Can you work these out from the model? Positions are in its coordinate system, mm. A direction names the side the tool comes from. Give positions to 0.01 mm unless a question says otherwise; leave off trailing zeros. Loops run counter-clockwise (first coordinate to the right, second up) from the corner with the lowest first, then second, coordinate; pieces in that order, holes last. Notation, with made-up numbers: (51, -21) - (74, -21) arc R25 ccw to (74, -4) - close; hole circle Ø5 at (18, -6). An arc over 180 degrees is marked (long way). Answer as a JSON object with one key per item and string values.
```python
from build123d import *

# Parameters (mm, degrees)
SKETCH1_R           = 16
BOSS_EXTRUDE1_DEPTH = 6
SKETCH2_R           = 21.5
SKETCH2_R_2         = 16
BOSS_EXTRUDE2_DEPTH = 23
CHAMFER1_SIZE       = 4
CHAMFER3_SIZE       = 1


with BuildPart() as part:
    # Sketch1 → Boss-Extrude1 (new body)
    with BuildSketch(Plane(origin=(0, 0, 0), x_dir=(1, 0, 0), z_dir=(0, 1, 0))):
        Polygon((38.105117767, 0), (19.052558883, 33), (-19.052558883, 33), (-38.105117767, 0), (-19.052558883, -33), (19.052558883, -33), align=None)
        with Locations(Location((0, 0, 0), (0, 0, 270))):
            Circle(SKETCH1_R, mode=Mode.SUBTRACT)
    extrude(amount=BOSS_EXTRUDE1_DEPTH)

    # Sketch2 → Boss-Extrude2 (add)
    with BuildSketch(Plane(origin=(0, 6, 0), x_dir=(1, 0, 0), z_dir=(0, 1, 0))):
        with Locations(Location((0, 0, 0), (0, 0, 270))):
            Circle(SKETCH2_R)
        with Locations(Location((0, 0, 0), (0, 0, 270))):
            Circle(SKETCH2_R_2, mode=Mode.SUBTRACT)
    extrude(amount=BOSS_EXTRUDE2_DEPTH)

    # Chamfer1
    chamfer1_edges = [part.edges().sort_by_distance(p)[0] for p in [
        (19.052558883, 3, 33),
        (-19.052558883, 3, 33),
        (-38.105117767, 3, 0),
        (-19.052558883, 3, -33),
        (19.052558883, 3, -33),
        (38.105117767, 3, 0),
    ]]
    chamfer(chamfer1_edges, length=CHAMFER1_SIZE)

    # Chamfer3
    chamfer3_edges = [part.edges().sort_by_distance(p)[0] for p in [
        (0, 6, -21.5),
        (-28.578838325, 6, 16.5),
        (-28.578838325, 6, -16.5),
        (28.578838325, 6, 16.5),
        (28.578838325, 6, -16.5),
        (0, 6, -33),
        (0, 6, 33),
        (-18.052558883, 6, -31.267949192),
        (18.052558883, 6, -31.267949192),
        (36.105117767, 6, 0),
        (18.052558883, 6, 31.267949192),
        (-18.052558883, 6, 31.267949192),
        (-36.105117767, 6, 0),
    ]]
    chamfer(chamfer3_edges, length=CHAMFER3_SIZE)


solid = part.part
```
1) Which directions (+Z, -Z, +X, -X, +Y, -Y) give clear straight access to the entire face, cutting with the end or side of a thin tool? Please do faces 1 (the cylindrical face through (14.531, 17.846, -15.846)), 2 (the flat face through (18.095, 2.465, 31.244)).
Check sheet entries:
{"face 1": "+Y", "face 2": "+Z, +X, +Y, -Y"}
2) Imagine slicing it at B-B on x = 0. Write out the boundary of the cut face in (y, z), and give its area (3 significant figures).
Check sheet entries:
{"outline": "(0, -33) - (5, -33) - (6, -32) - (6, -22.5) - (7, -21.5) - (29, -21.5) - (29, -16) - (0, -16) - close; (0, 16) - (29, 16) - (29, 21.5) - (7, 21.5) - (6, 22.5) - (6, 32) - (5, 33) - (0, 33) - close", "area": "457 mm2"}
3) I need wall thicknesses on L1, parallel to Z at x = 0.5, y = 7.25; L2, parallel to X at y = 7.75, z = 0; L3, parallel to Y at x = -10.5, z = 25. Which ranges of each line are inside material? Lowest first, please.
Check sheet entries:
{"L1": "-21.49 to -15.99, 15.99 to 21.49", "L2": "-21.5 to -16, 16 to 21.5", "L3": "0 to 6"}
4) Imagine slicing it at D-D on z = 26. Write out the boundary of the cut face in (x, y), and give its area (3 significant figures).
Check sheet entries:
{"outline": "(-23.09, 0) - (23.09, 0) - (23.09, 5) - (21.94, 6) - (-21.94, 6) - (-23.09, 5) - close", "area": "276 mm2"}
5) Imagine slicing it at C-C on y = 3.75. Write out the boundary of the cut face in (x, z).
Check sheet entries:
{"outline": "(-36.11, -3.46) - (-21.05, -29.54) - (-15.05, -33) - (15.05, -33) - (21.05, -29.54) - (36.11, -3.46) - (36.11, 3.46) - (21.05, 29.54) - (15.05, 33) - (-15.05, 33) - (-21.05, 29.54) - (-36.11, 3.46) - close; hole circle Ø32 at (0, 0)"}
6) Imagine slicing it at A-A on z = 0. Write out the boundary of the cut face in (x, y).
Check sheet entries:
{"outline": "(-36.11, 0) - (-16, 0) - (-16, 29) - (-21.5, 29) - (-21.5, 7) - (-22.5, 6) - (-35.11, 6) - (-36.11, 5) - close; (16, 0) - (36.11, 0) - (36.11, 5) - (35.11, 6) - (22.5, 6) - (21.5, 7) - (21.5, 29) - (16, 29) - close"}
7) I'm going to push flat-ended pins straight in: P1, Ø6, axis at x = 7, y = 8.5, coming from the -Z side; P2, Ø1.5, axis at y = 17.5, z = 13.5, coming from the +X side; P3, Ø12, axis at x = 21.5, y = 6.5, coming from the +Z side. Where does each tip first touch, or does it pass through?
Check sheet entries:
{"P1": "z = -32.5", "P2": "x = 17.31", "P3": "z = 32.63"}
